Input: dimensioned drawing with shaded views. Units: mm. Origin: part minimum x, y, z. A direction names the side the tool comes from. Give positions to 0.01 mm unless a question says otherwise; leave off trailing zeros. Loops run counter-clockwise (first coordinate to the right, second up) from the corner with the lowest first, then second, coordinate; pieces in that order, holes last.
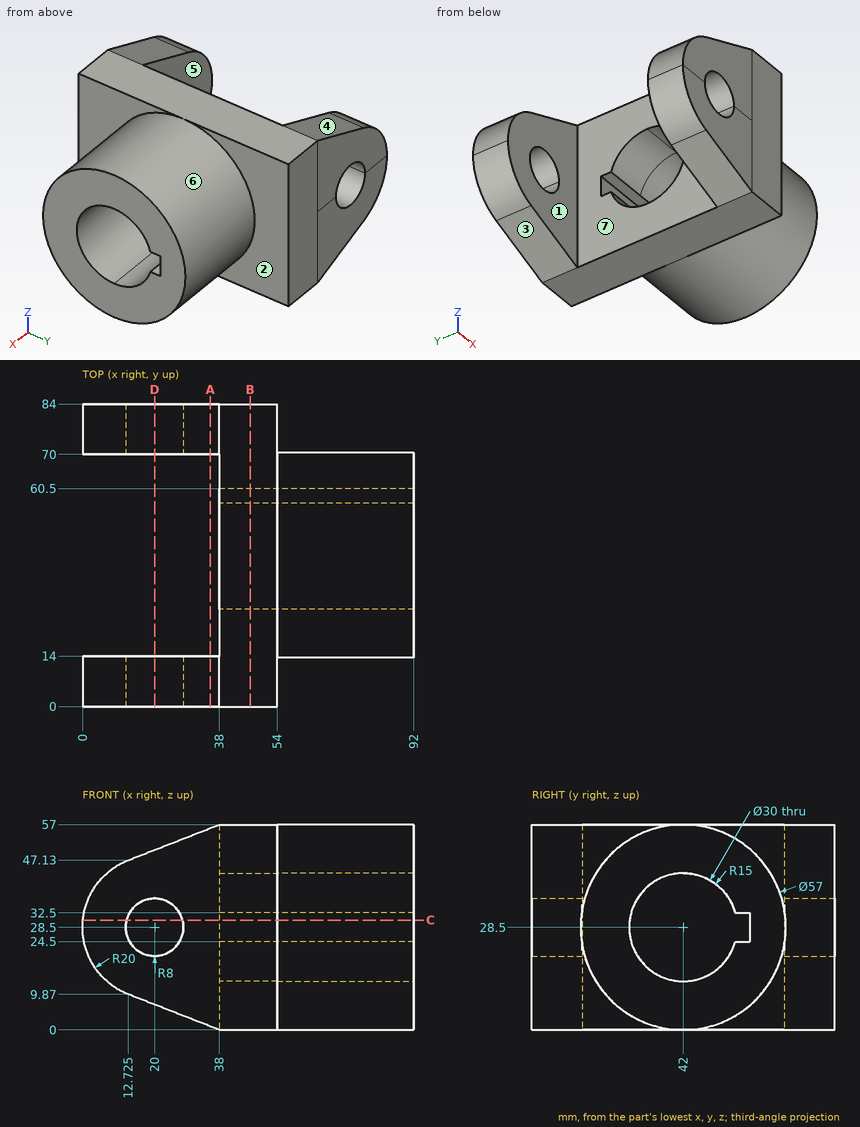
Item 1: Section query A-A on x = 35.5. Return loops of the section in (y, z), plus the area to 3 significant figures.
Values follow:
outline: (0, 0.98) - (14, 0.98) - (14, 56.02) - (0, 56.02) - close; (70, 0.98) - (84, 0.98) - (84, 56.02) - (70, 56.02) - close
area: 1,540 mm2
Item 2: Section query D-D on x = 20. Return loops of the section in (y, z).
Values follow:
outline: (0, 7.03) - (14, 7.03) - (14, 20.5) - (0, 20.5) - close; (0, 36.5) - (14, 36.5) - (14, 49.97) - (0, 49.97) - close; (70, 7.03) - (84, 7.03) - (84, 20.5) - (70, 20.5) - close; (70, 36.5) - (84, 36.5) - (84, 49.97) - (70, 49.97) - close
Item 3: Draft query along Y for the marked faces 4, 5, 6 and 7. Return one class per face: +Y half, -Y half, draft (parallel to the pull), parting line (faces both ways), or undercut.
Values follow:
face 4: draft
face 5: undercut
face 6: parting line
face 7: undercut
Item 4: Section query C-C on z = 30.5. Return loops of the section in (x, y).
Values follow:
outline: (0.1, 0) - (12.25, 0) - (12.25, 14) - (0.1, 14) - close; (0.1, 70) - (12.25, 70) - (12.25, 84) - (0.1, 84) - close; (27.75, 0) - (54, 0) - (54, 13.57) - (92, 13.57) - (92, 27.13) - (38, 27.13) - (38, 14) - (27.75, 14) - close; (27.75, 70) - (38, 70) - (38, 60.5) - (92, 60.5) - (92, 70.43) - (54, 70.43) - (54, 84) - (27.75, 84) - close
Item 5: Ray query, probe 1 along Y at (x, z) = (36, 22); probe 2 along Y at (x, z) = (82, 28.5); probe 3 along Z at (x, y) = (44, 42). Return the intervals inside material, ascending.
Values follow:
probe 1: y = 0 to 14, 70 to 84
probe 2: y = 13.5 to 27, 60.5 to 70.5
probe 3: z = 0 to 13.5, 43.5 to 57
Item 6: Set-up query: the marked faces 1, 2 and 3. Return all of +Z, -Z, +X, -X, +Y, -Y with unobstructed straight access to the full face (end or side cutting, diameter ignored); none if empty.
Values follow:
face 1: +Z, -Z, -X
face 2: +X, +Y
face 3: -Z, -X, +Y, -Y
Item 7: Section query B-B on x = 46.5. Return loops of the section in (y, z), plus the area to 3 significant figures.
Values follow:
outline: (0, 0) - (84, 0) - (84, 57) - (0, 57) - close; hole (56.46, 24.5) - (60.5, 24.5) - (60.5, 32.5) - (56.46, 32.5) arc R15 ccw (long way) to start
area: 4,050 mm2
Item 8: Pin query (flat end, axial travel): pin 1 (1.5 mm diameter, centred on x = 63, z = 15, fed in from +Y); pin 2 (1.5 mm diameter, centred on x = 78.5, y = 51.5, fed in from +Z); pin 3 (4 mm diameter, centred on x = 75.5, z = 27.5, fed in from -Y). Return the tip coordinate at first contact, or that it passes through.
Values follow:
pin 1: stops at y = 67.49
pin 2: stops at z = 55.62
pin 3: stops at y = 13.5
